from build123d import *

# Parameters (mm, degrees)
F0_R     = 11
F0_R_2   = 7.5
F1_DEPTH = 2
F0_R_3   = 4.175
F2_DEPTH = 3
F3_DEPTH = 5.5
F4_R     = 0.99999


# Not quite as in the source:
# - a fillet or chamfer is up to 0.001 mm smaller than in the source, because OpenCascade refuses the exact size


with BuildPart() as f1:
    # F0 (on Top) → F1 (new body)
    with BuildSketch(Plane.XY):
        Circle(F0_R)
        Circle(F0_R_2, mode=Mode.SUBTRACT)
    extrude(amount=F1_DEPTH)

    # F0 (on Top) → F2 (join)
    with BuildSketch(Plane.XY):
        Circle(F0_R_2)
        Circle(F0_R_3, mode=Mode.SUBTRACT)
    extrude(amount=F2_DEPTH)

    # F0 (on Top) → F3 (join)
    with BuildSketch(Plane.XY):
        Circle(F0_R_3)
    extrude(amount=F3_DEPTH)

    # F4 (radius 1 in the source; OpenCascade refuses exactly that, so slightly less here)
    f4_edges = [f1.edges().sort_by_distance(p)[0] for p in [
        (-11, 0, 2),
        (-11, 0, 0),
    ]]
    fillet(f4_edges, radius=F4_R)


solid = f1.part
Could you check a few things on this model? Use its own coordinates, in mm. A direction names the side the tool comes from. Give positions to 0.01 mm unless a question says otherwise; leave off trailing zeros. Write each loop counter-clockwise with the first axis right and the second up, starting at its lowest first coordinate (ties: lowest second). Pieces come first, ordered by that corner, then holes. Notation, with made-up numbers: (0, 1.5) - (16, 1.5) arc R37 ccw to (16, 38.5) - close; hole circle Ø10 at (68, 51.25). An arc over 180 degrees is marked (long way). Use CSV: the item, a comma, the result in double quotes. Start each with the question number.
Item 1: I'm going to push flat-ended pins straight in: pin 1 (8 mm diameter, centred on x = -0.5, y = -6, fed in from -Z); pin 2 (2 mm diameter, centred on x = -7, z = 0.5, fed in from +Y). Where does each tip first touch, or does it pass through?
Item 2: I want a section at C-C, the plane z = 4.2. Please give me the cut outline in (x, y) (3 decimals).
Item 3: For faces 1 (the face through (3.2, -3.2, 3)), 2 (the face through (0, 0, 5.5)), which set-ups out of +Z, -Z, +X, -X, +Y, -Y let a thin tool reach every point of the face, with its end or its side?
Item 4: I want a section at D-D, the plane z = 0.4. Please give me the cut outline in (x, y), then the cut area to 3 significant figures.
Item 5: If I drill on line 1 along Z through (x, y) = (-7, -3.5); line 2 along Z through (x, y) = (-1, 7.25); line 3 along Y through (x, z) = (4, 2.4), over which ranges is the centre line in solid material (lowest first)?
Findings:
1,pin 1,"stops at z = 0"
1,pin 2,"stops at y = 9.17"
2,outline,"circle Ø8.35 at (0, 0)"
3,face 1,"+Z"
3,face 2,"+Z, +X, -X, +Y, -Y"
4,outline,"circle Ø21.6 at (0, 0)"
4,area,"366 mm2"
5,line 1,"z = 0 to 2"
5,line 2,"z = 0 to 3"
5,line 3,"y = -6.34 to 6.34"
